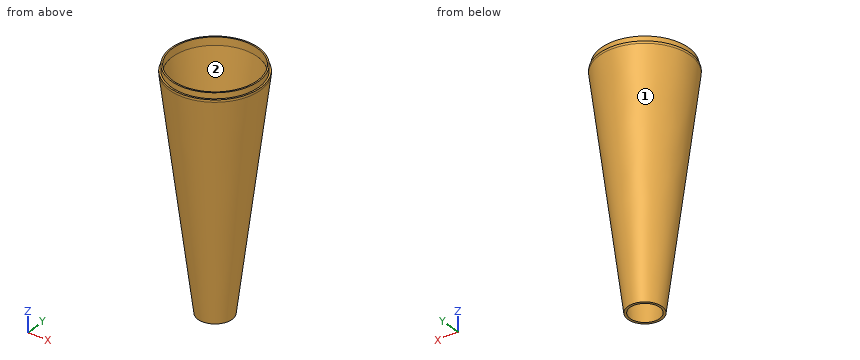
from build123d import *

# Parameters (mm, degrees)
F0_R      = 40
F1_DEPTH  = 2
F2_R      = 38.5
F3_DEPTH  = 5
F7_R      = 15
F4_R      = 40
F9_T      = -2
F10_R     = 37.2180973158
F11_DEPTH = 7.001


with BuildPart() as f1:
    # F0 (on Top) → F1 (new body)
    with BuildSketch(Plane.XY):
        Circle(F0_R)
    extrude(amount=F1_DEPTH)

    # F2 (on face) → F3 (join)
    with BuildSketch(Plane.XY.offset(2)):
        Circle(F2_R)
    extrude(amount=F3_DEPTH)

    # F7 (on plane+point) → F8 section 0
    with BuildSketch(Plane.XY.offset(-200)):
        Circle(F7_R)
    # F4 (on face) → F8 section 1
    with BuildSketch(Plane(origin=(0, 0, 0), x_dir=(1, 0, 0), z_dir=(0, 0, -1))):
        Circle(F4_R)
    loft()

    # F9
    f9_openings = [f1.faces().sort_by_distance(p)[0] for p in [
        (0, 0, -200),
    ]]
    offset(amount=F9_T, openings=f9_openings, kind=Kind.INTERSECTION)

    # F10 (on face) → F11 (cut, through all)
    with BuildSketch(Plane.XY.offset(7)):
        Circle(F10_R)
    extrude(amount=-F11_DEPTH, mode=Mode.SUBTRACT)


solid = f1.part
Input: part model. Units: mm. Frame: model coordinates. Face numbers are marked on the shaded views. Give positions to 0.01 mm unless a question says otherwise; leave off trailing zeros. Write each loop counter-clockwise with the first axis right and the second up, starting at its lowest first coordinate (ties: lowest second). Pieces come first, ordered by that corner, then holes.
Q1. Pull-direction query (X, two-part tool) for the marked faces 1 and 2; classes: pulls with the +X half, pulls with the -X half, needs draft (parallel to the pull), parting line crosses it, or undercut.
Q2. First-contact query: P1, Ø5, axis at x = 5.5, z = -95.5, coming from the +Y side; P2, Ø3, axis at x = 22, z = -85, coming from the +Y side; P3, Ø12, axis at x = 21.5, z = -60, coming from the +Y side. Flat tips, straight axial feed; report the tip coordinate or a pass-through.
Q3. Section C-C, the plane z = -24. Output: boundary loops of the cut face in (x, y), plus the area to 3 significant figures.
Q4. Section A-A, the plane x = 0. Output: boundary loops of the cut face in (y, z).
Q5. Section B-B, the plane z = -126.5. Output: boundary loops of the cut face in (x, y) (1 decimal), plus the area to 3 significant figures.
Q6. Material intervals for probe 1 along Y at (x, z) = (0, 2.25); probe 2 along X at (y, z) = (-26, -19); probe 3 along Y at (x, z) = (22, -17.5), sorted ascending.
Filled in:
1. face 1: parting line crosses it
1. face 2: undercut
2. P1: stops at y = 28.04
2. P2: stops at y = 21.06
2. P3: stops at y = 28.68
3. outline: circle Ø74 at (0, 0); hole circle Ø69.97 at (0, 0)
3. area: 456 mm2
4. outline: (-40, 0) - (-15, -200) - (-12.98, -200) - (-37.98, 0) - (-37.22, 0) - (-37.22, 7) - (-38.5, 7) - (-38.5, 2) - (-40, 2) - close; (12.98, -200) - (15, -200) - (40, 0) - (40, 2) - (38.5, 2) - (38.5, 7) - (37.22, 7) - (37.22, 0) - (37.98, 0) - close
5. outline: circle Ø48.4 at (0, 0); hole circle Ø44.3 at (0, 0)
5. area: 294 mm2
6. probe 1: y = -38.5 to -37.22, 37.22 to 38.5
6. probe 2: x = -27.2 to -24.33, 24.33 to 27.2
6. probe 3: y = -30.75 to -28.24, 28.24 to 30.75
